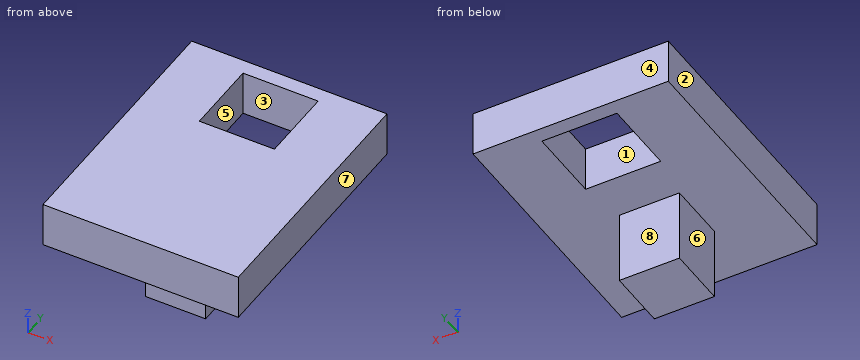
from build123d import *

# Parameters (mm, degrees)
SKETCH1_W           = 41.275
SKETCH1_H           = 53.975
SKETCH1_W_2         = 15.875
SKETCH1_H_2         = 15.875
BOSS_EXTRUDE1_DEPTH = 9.525
SKETCH2_W           = 12.7
SKETCH2_H           = 12.7
BOSS_EXTRUDE2_DEPTH = 15.477083255


with BuildPart() as part:
    # Sketch1 → Boss-Extrude1 (new body)
    with BuildSketch(Plane.XY):
        with Locations((-6.943541269, -10.118279033)):
            Rectangle(SKETCH1_W, SKETCH1_H)
        with Locations((-6.943541269, 5.756720967)):
            Rectangle(SKETCH1_W_2, SKETCH1_H_2, mode=Mode.SUBTRACT)
    extrude(amount=-BOSS_EXTRUDE1_DEPTH)

    # Sketch2 → Boss-Extrude2 (add)
    with BuildSketch(Plane(origin=(0, 0, -9.525), x_dir=(-1, 0, 0), z_dir=(0, 0, -1))):
        with Locations((6.943541269, -18.055779033)):
            Rectangle(SKETCH2_W, SKETCH2_H)
    extrude(amount=BOSS_EXTRUDE2_DEPTH)


solid = part.part
CAD build for the part. Positions are in the model's coordinates, mm. Face numbers are marked on the shaded views. A direction names the side the tool comes from. Give positions to 0.01 mm unless a question says otherwise; leave off trailing zeros. Loops run counter-clockwise (first coordinate to the right, second up) from the corner with the lowest first, then second, coordinate; pieces in that order, holes last. Notation, with made-up numbers: M 45,73 L 91,73 A32 cw 91,104 Z; hole C -0.75,29.25 d10. An arc over 180 degrees is marked long. Answer in a Markdown table with one row per item. Add a question column.
Item 1: Probe probe 1 along X at (y, z) = (12.5, -9); probe 2 along Y at (x, z) = (-9, -22); probe 3 along Z at (x, y) = (6.5, -19) (3 decimals). List the from-to ranges inside material, lowest first.
Item 2: Mould opens along Y. For the marked faces 1, 2, 3 and 4 say: +Y half, -Y half, draft (parallel to the pull), parting line (faces both ways), or undercut.
Item 3: Band-saw the part on A-A on y = -0.5. Give the cut face in (x, z) (3 decimals), then the cut area to 3 significant figures.
Item 4: Band-saw the part on B-B on x = -7. Give the cut face in (y, z) (3 decimals).
Item 5: Drop flat-ended pins along their axis: P1, Ø10, axis at x = -8.5, z = -19.5, coming from the +Y side; P2, Ø2, axis at x = -9, y = -15, coming from the +Z side; P3, Ø2, axis at x = -11, z = -11.5, coming from the -Y side; P4, Ø6.5, axis at y = -21, z = -19.5, coming from the +X side. Give the stop position or say it passes through.
Item 6: Tool access for the marked faces 5, 6, 7 and 8: list every direction of +Z, -Z, +X, -X, +Y, -Y with a clear straight run to the whole face (end or side of a thin tool).
Item 7: Band-saw the part on C-C on z = -4. Give the cut face in (x, y), then the cut area to 3 significant figures.
Item 8: Band-saw the part on D-D on x = -25. Give the cut face in (y, z) (3 decimals).
Reply:
| question | item | result |
|---|---|---|
| 1 | probe 1 | x = -27.58 to -14.88, 0.99 to 13.69 |
| 1 | probe 2 | y = -24.41 to -11.71 |
| 1 | probe 3 | z = -9.525 to 0 |
| 2 | face 1 | undercut |
| 2 | face 2 | draft |
| 2 | face 3 | undercut |
| 2 | face 4 | +Y half |
| 3 | outline | M -27.581,-9.525 L -14.881,-9.525 L -14.881,0 L -27.581,0 Z; M 0.994,-9.525 L 13.694,-9.525 L 13.694,0 L 0.994,0 Z |
| 3 | area | 242 mm^2 |
| 4 | outline | M -37.106,-9.525 L -24.406,-9.525 L -24.406,-25.002 L -11.706,-25.002 L -11.706,-9.525 L -2.181,-9.525 L -2.181,0 L -37.106,0 Z; M 13.694,-9.525 L 16.869,-9.525 L 16.869,0 L 13.694,0 Z |
| 5 | P1 | stops at y = -11.71 |
| 5 | P2 | stops at z = 0 |
| 5 | P3 | stops at y = -24.41 |
| 5 | P4 | stops at x = -0.59 |
| 6 | face 5 | +Z, -Z |
| 6 | face 6 | -Z, -X, +Y, -Y |
| 6 | face 7 | +Z, -Z, +X, +Y, -Y |
| 6 | face 8 | -Z, +X, -X, +Y |
| 7 | outline | M -27.58,-37.11 L 13.69,-37.11 L 13.69,16.87 L -27.58,16.87 Z; hole M -14.88,-2.18 L 0.99,-2.18 L 0.99,13.69 L -14.88,13.69 Z |
| 7 | area | 1,980 mm^2 |
| 8 | outline | M -37.106,-9.525 L 16.869,-9.525 L 16.869,0 L -37.106,0 Z |
